Read the model definition and answer for the solid it produces. Units are mm, in the model's axes. A direction names the side the tool comes from. Coordinates: 2 decimals unless noted, no trailing zeros. Write each loop counter-clockwise with the first axis right and the second up, starting at its lowest first coordinate (ties: lowest second). Pieces come first, ordered by that corner, then holes.
(1) Section C-C on z = 18 is taken. Write down the section's boundary in (x, y).
(2) Which of the six approach directions +Z, -Z, +X, -X, +Y, -Y give full straight-line access (tool end or side, diameter ignored) to faces 3 (the flat face through (46.571, 0.986, 9.376)), 4 (the flat face through (35.5, 13.47, 4.01)), 5 (the cylindrical face through (46.095, 20.54, 1.521))?
(3) Given pin 1 (4.5 mm diameter, centred on x = 19.5, y = 13.5, fed in from +Z); pin 2 (5.5 mm diameter, centred on x = 48, y = 12, fed in from +Z); pin 3 (8 mm diameter, centred on x = 8, z = 15, fed in from +Y), each flat-ended and moving along its own axis, determine where each tip first touches the part or whether it passes through.
(4) Find the intervals of material crossed by probe 1 along Y at (x, z) = (38, 0.85); probe 2 along Z at (x, y) = (8, 3.4); probe 3 along Z at (x, y) = (28, 4.25), in increasing order.
(5) Section B-B on z = 1.5 is taken. State how many separate pieces and enclosed holes the cut face has, then the cut area to 3 significant figures.
(6) Section D-D on z = 6.5 is taken. Write down the section's boundary in (x, y), then the cut area to 3 significant figures.
(7) Section A-A on x = 43 is taken. Write down the section's boundary in (y, z), then the cut area to 3 significant figures.
(8) The mould has two halves that part along X. Classify faces 1 (the flat face through (16.573, 0.986, 9.524)), 2 (the flat face through (31, 30, 2)): +X half, -X half, draft (parallel to the pull), parting line (faces both ways), or undercut.
from build123d import *

# Parameters (mm, degrees)
SKETCH_1_W                  = 66
SKETCH_1_H                  = 30
EXTRUDE_1_DEPTH             = 20
SKETCH_2_W                  = 15
SKETCH_2_H                  = 25
CUT_EXTRUDE_1_DEPTH         = 67
CUT_EXTRUDE_2_DEPTH         = 2
CUT_EXTRUDE_3_DEPTH         = 2
CUT_EXTRUDE_4_DEPTH         = 2
CUT_EXTRUDE_5_DEPTH         = 2
CUT_EXTRUDE_6_DEPTH         = 2
CUT_EXTRUDE_7_DEPTH         = 2
CUT_EXTRUDE_8_DEPTH         = 2
CUT_EXTRUDE_9_DEPTH         = 2
CUT_EXTRUDE_10_DEPTH        = 2
CUT_EXTRUDE_11_DEPTH        = 2
CUT_EXTRUDE_12_DEPTH        = 2
CUT_EXTRUDE_13_DEPTH        = 2
CUT_EXTRUDE_14_DEPTH        = 2
CUT_EXTRUDE_15_DEPTH        = 2
CUT_EXTRUDE_16_DEPTH        = 2
CUT_EXTRUDE_17_DEPTH        = 2
CUT_EXTRUDE_18_DEPTH        = 2
CUT_EXTRUDE_19_DEPTH        = 2
HOLE_WIZARD_3_0_3_1_D       = 3
HOLE_WIZARD_3_0_3_1_DEPTH   = 5
HOLE_WIZARD_3_3_3_3_1_D     = 3.3
HOLE_WIZARD_3_3_3_3_1_DEPTH = 5
HOLE_WIZARD_3_5_3_5_1_D     = 3.5
HOLE_WIZARD_3_5_3_5_1_DEPTH = 5
HOLE_WIZARD_3_8_3_8_1_D     = 3.8
HOLE_WIZARD_3_8_3_8_1_DEPTH = 20
HOLE_WIZARD_4_5_4_5_1_D     = 4.5
HOLE_WIZARD_4_5_4_5_1_DEPTH = 20
HOLE_WIZARD_3_5_3_5_2_D     = 3.5
HOLE_WIZARD_3_5_3_5_2_DEPTH = 20
HOLE_WIZARD_4_8_4_8_1_D     = 4.8
HOLE_WIZARD_4_8_4_8_1_DEPTH = 20
HOLE_WIZARD_3_3_3_3_2_D     = 3.3
HOLE_WIZARD_3_3_3_3_2_DEPTH = 20
CHAMFER_1_SIZE              = 5
FILLET_1_R                  = 3
FILLET_2_R                  = 5


with BuildPart() as part:
    # 草图1 → 凸台-拉伸1 (new body)
    with BuildSketch(Plane(origin=(0, 0, 0), x_dir=(-1, 0, 0), z_dir=(0, 0, -1))):
        with Locations((-33, 15)):
            Rectangle(SKETCH_1_W, SKETCH_1_H)
    extrude(amount=-EXTRUDE_1_DEPTH)

    # 草图2 → 切除-拉伸1 (cut, through all)
    with BuildSketch(Plane.ZY):
        with Locations((12.5, 17.5)):
            Rectangle(SKETCH_2_W, SKETCH_2_H)
    extrude(amount=-CUT_EXTRUDE_1_DEPTH, mode=Mode.SUBTRACT)

    # 草图3 → 切除-拉伸2 (cut)
    with BuildSketch(Plane.XZ):
        Polygon((58.142658315, 8.502908551), (61.099899192, 10.375), (60.957240877, 13.872091449), (57.857341685, 15.497091449), (54.900100808, 13.625), (55.042759123, 10.127908551), align=None)
    extrude(amount=-CUT_EXTRUDE_2_DEPTH, mode=Mode.SUBTRACT)

    # 草图4 → 切除-拉伸3 (cut)
    with BuildSketch(Plane.XZ):
        Polygon((48.114375157, 8.551896416), (51.043332877, 10.375), (50.92895772, 13.823103584), (47.885624843, 15.448103584), (44.956667123, 13.625), (45.07104228, 10.176896416), align=None)
    extrude(amount=-CUT_EXTRUDE_3_DEPTH, mode=Mode.SUBTRACT)

    # 草图5 → 切除-拉伸4 (cut)
    with BuildSketch(Plane.XZ):
        Polygon((38.085974854, 8.601087185), (40.98653227, 10.375), (40.900557416, 13.773912815), (37.914025146, 15.398912815), (35.01346773, 13.625), (35.099442584, 10.226087185), align=None)
    extrude(amount=-CUT_EXTRUDE_4_DEPTH, mode=Mode.SUBTRACT)

    # 草图6 → 切除-拉伸5 (cut)
    with BuildSketch(Plane.XZ):
        Polygon((28.05745059, 8.650492659), (30.929483743, 10.375), (30.872033153, 13.724507341), (27.94254941, 15.349507341), (25.070516257, 13.625), (25.127966847, 10.275492659), align=None)
    extrude(amount=-CUT_EXTRUDE_5_DEPTH, mode=Mode.SUBTRACT)

    # 草图7 → 切除-拉伸6 (cut)
    with BuildSketch(Plane.XZ):
        Polygon((18.02879498, 8.700125631), (20.872172523, 10.375), (20.843377542, 13.674874369), (17.97120502, 15.299874369), (15.127827477, 13.625), (15.156622458, 10.325125631), align=None)
    extrude(amount=-CUT_EXTRUDE_6_DEPTH, mode=Mode.SUBTRACT)

    # 草图8 → 切除-拉伸7 (cut)
    with BuildSketch(Plane.XZ):
        Polygon((8, 8.75), (10.814582562, 10.375), (10.814582562, 13.625), (8, 15.25), (5.185417438, 13.625), (5.185417438, 10.375), align=None)
    extrude(amount=-CUT_EXTRUDE_7_DEPTH, mode=Mode.SUBTRACT)

    # 草图9 → 切除-拉伸8 (cut)
    with BuildSketch(Plane.XY.offset(5)):
        Polygon((10.05, 18.449295844), (12.1, 22), (10.05, 25.550704156), (5.95, 25.550704156), (3.9, 22), (5.95, 18.449295844), align=None)
    extrude(amount=-CUT_EXTRUDE_8_DEPTH, mode=Mode.SUBTRACT)

    # 草图10 → 切除-拉伸9 (cut)
    with BuildSketch(Plane.XY.offset(5)):
        Polygon((9.6, 9.228718708), (11.2, 12), (9.6, 14.771281292), (6.4, 14.771281292), (4.8, 12), (6.4, 9.228718708), align=None)
    extrude(amount=-CUT_EXTRUDE_9_DEPTH, mode=Mode.SUBTRACT)

    # 草图11 → 切除-拉伸10 (cut)
    with BuildSketch(Plane.XY.offset(5)):
        Polygon((19.625, 9.185417438), (21.25, 12), (19.625, 14.814582562), (16.375, 14.814582562), (14.75, 12), (16.375, 9.185417438), align=None)
    extrude(amount=-CUT_EXTRUDE_10_DEPTH, mode=Mode.SUBTRACT)

    # 草图12 → 切除-拉伸11 (cut)
    with BuildSketch(Plane.XY.offset(5)):
        Polygon((29.65, 9.142116168), (31.3, 12), (29.65, 14.857883832), (26.35, 14.857883832), (24.7, 12), (26.35, 9.142116168), align=None)
    extrude(amount=-CUT_EXTRUDE_11_DEPTH, mode=Mode.SUBTRACT)

    # 草图13 → 切除-拉伸12 (cut)
    with BuildSketch(Plane.XY.offset(5)):
        Polygon((20.075, 18.405994574), (22.15, 22), (20.075, 25.594005426), (15.925, 25.594005426), (13.85, 22), (15.925, 18.405994574), align=None)
    extrude(amount=-CUT_EXTRUDE_12_DEPTH, mode=Mode.SUBTRACT)

    # 草图14 → 切除-拉伸13 (cut)
    with BuildSketch(Plane.XY.offset(5)):
        Polygon((30.1, 18.362693304), (32.2, 22), (30.1, 25.637306696), (25.9, 25.637306696), (23.8, 22), (25.9, 18.362693304), align=None)
    extrude(amount=-CUT_EXTRUDE_13_DEPTH, mode=Mode.SUBTRACT)

    # 草图15 → 切除-拉伸14 (cut)
    with BuildSketch(Plane.XY.offset(5)):
        Polygon((40.125, 18.319392034), (42.25, 22), (40.125, 25.680607966), (35.875, 25.680607966), (33.75, 22), (35.875, 18.319392034), align=None)
    extrude(amount=-CUT_EXTRUDE_14_DEPTH, mode=Mode.SUBTRACT)

    # 草图16 → 切除-拉伸15 (cut)
    with BuildSketch(Plane.XY.offset(5)):
        Polygon((50.15, 18.276090764), (52.3, 22), (50.15, 25.723909236), (45.85, 25.723909236), (43.7, 22), (45.85, 18.276090764), align=None)
    extrude(amount=-CUT_EXTRUDE_15_DEPTH, mode=Mode.SUBTRACT)

    # 草图17 → 切除-拉伸16 (cut)
    with BuildSketch(Plane.XY.offset(5)):
        Polygon((60.175, 18.232789494), (62.35, 22), (60.175, 25.767210506), (55.825, 25.767210506), (53.65, 22), (55.825, 18.232789494), align=None)
    extrude(amount=-CUT_EXTRUDE_16_DEPTH, mode=Mode.SUBTRACT)

    # 草图18 → 切除-拉伸17 (cut)
    with BuildSketch(Plane.XY.offset(5)):
        Polygon((59.725, 9.012212357), (61.45, 12), (59.725, 14.987787643), (56.275, 14.987787643), (54.55, 12), (56.275, 9.012212357), align=None)
    extrude(amount=-CUT_EXTRUDE_17_DEPTH, mode=Mode.SUBTRACT)

    # 草图19 → 切除-拉伸18 (cut)
    with BuildSketch(Plane.XY.offset(5)):
        Polygon((49.7, 9.055513627), (51.4, 12), (49.7, 14.944486373), (46.3, 14.944486373), (44.6, 12), (46.3, 9.055513627), align=None)
    extrude(amount=-CUT_EXTRUDE_18_DEPTH, mode=Mode.SUBTRACT)

    # 草图20 → 切除-拉伸19 (cut)
    with BuildSketch(Plane.XY.offset(5)):
        Polygon((39.675, 9.098814897), (41.35, 12), (39.675, 14.901185103), (36.325, 14.901185103), (34.65, 12), (36.325, 9.098814897), align=None)
    extrude(amount=-CUT_EXTRUDE_19_DEPTH, mode=Mode.SUBTRACT)

    # Ø3.0 (3) 直径孔1
    with Locations(Plane(origin=(0, 5, 0), x_dir=(1, 0, 0), z_dir=(0, 1, 0))):
        with Locations((8, -12)):
            Hole(HOLE_WIZARD_3_0_3_1_D / 2, depth=HOLE_WIZARD_3_0_3_1_DEPTH)

    # Ø3.3 (3.3) 直径孔1
    with Locations(Plane(origin=(0, 5, 0), x_dir=(1, 0, 0), z_dir=(0, 1, 0))):
        with Locations((38, -12), (28, -12), (18, -12)):
            Hole(HOLE_WIZARD_3_3_3_3_1_D / 2, depth=HOLE_WIZARD_3_3_3_3_1_DEPTH)

    # Ø3.5 (3.5) 直径孔1
    with Locations(Plane(origin=(0, 5, 0), x_dir=(1, 0, 0), z_dir=(0, 1, 0))):
        with Locations((58, -12), (48, -12)):
            Hole(HOLE_WIZARD_3_5_3_5_1_D / 2, depth=HOLE_WIZARD_3_5_3_5_1_DEPTH)

    # Ø3.8 (3.8) 直径孔1
    with Locations(Plane(origin=(0, 0, 0), x_dir=(-1, 0, 0), z_dir=(0, 0, -1))):
        with Locations((-58, 12)):
            Hole(HOLE_WIZARD_3_8_3_8_1_D / 2, depth=HOLE_WIZARD_3_8_3_8_1_DEPTH)

    # Ø4.5 (4.5) 直径孔1
    with Locations(Plane(origin=(0, 0, 0), x_dir=(-1, 0, 0), z_dir=(0, 0, -1))):
        with Locations((-28, 22), (-18, 22), (-8, 22)):
            Hole(HOLE_WIZARD_4_5_4_5_1_D / 2, depth=HOLE_WIZARD_4_5_4_5_1_DEPTH)

    # Ø3.5 (3.5) 直径孔2
    with Locations(Plane(origin=(0, 0, 0), x_dir=(-1, 0, 0), z_dir=(0, 0, -1))):
        with Locations((-28, 12), (-38, 12), (-48, 12)):
            Hole(HOLE_WIZARD_3_5_3_5_2_D / 2, depth=HOLE_WIZARD_3_5_3_5_2_DEPTH)

    # Ø4.8 (4.8) 直径孔1
    with Locations(Plane(origin=(0, 0, 0), x_dir=(-1, 0, 0), z_dir=(0, 0, -1))):
        with Locations((-58, 22), (-48, 22), (-38, 22)):
            Hole(HOLE_WIZARD_4_8_4_8_1_D / 2, depth=HOLE_WIZARD_4_8_4_8_1_DEPTH)

    # Ø3.3 (3.3) 直径孔2
    with Locations(Plane(origin=(0, 0, 0), x_dir=(-1, 0, 0), z_dir=(0, 0, -1))):
        with Locations((-8, 12), (-18, 12)):
            Hole(HOLE_WIZARD_3_3_3_3_2_D / 2, depth=HOLE_WIZARD_3_3_3_3_2_DEPTH)

    # 倒角1
    chamfer_1_edges = [part.edges().sort_by_distance(p)[0] for p in [
        (66, 30, 2.5),
    ]]
    chamfer(chamfer_1_edges, length=CHAMFER_1_SIZE)

    # 圆角1
    fillet_1_edges = [part.edges().sort_by_distance(p)[0] for p in [
        (33, 5, 5),
    ]]
    fillet(fillet_1_edges, radius=FILLET_1_R)

    # 圆角2
    fillet_2_edges = [part.edges().sort_by_distance(p)[0] for p in [
        (0, 2.5, 20),
    ]]
    fillet(fillet_2_edges, radius=FILLET_2_R)


solid = part.part
Response:
1. outline: (1, 0) - (66, 0) - (66, 5) - (1, 5) - close
2. face 3: -Y
2. face 4: +Z
2. face 5: +Z, -Z
3. pin 1: stops at z = 5
3. pin 2: stops at z = 3
3. pin 3: stops at y = 5
4. probe 1: y = 0 to 10.25, 13.75 to 19.6, 24.4 to 30
4. probe 2: z = 0 to 10.5, 13.5 to 20
4. probe 3: z = 0 to 10.35, 13.65 to 20
5. separate pieces: 1
5. enclosed holes: 12
5. area: 1,810 mm2
6. outline: (0, 0) - (66, 0) - (66, 5.4) - (0, 5.4) - close
6. area: 357 mm2
7. outline: (0, 0) - (30, 0) - (30, 5) - (8, 5) arc R3 cw to (5, 8) - (5, 20) - (0, 20) - close
7. area: 227 mm2
8. face 1: undercut
8. face 2: draft
